The model under review builds one solid part; all positions refer to its coordinate system, in mm. A direction names the side the tool comes from. Coordinates: 2 decimals unless noted, no trailing zeros. Write each loop counter-clockwise with the first axis right and the second up, starting at its lowest first coordinate (ties: lowest second). Pieces come first, ordered by that corner, then holes. Notation, with made-up numbers: M 1,32 L 59,32 A23 cw 59,48 Z; hole C 43.25,6.5 d9. An arc over 180 degrees is marked long. Answer as a JSON object with one key per item and string values.
```python
from build123d import *

# Parameters (mm, degrees)
F0_W          = 310
F0_H          = 200
F1_DEPTH      = 15
F3_R          = 10
F2_R          = 6.5
F4_DEPTH      = 4
F4_DEPTH_BACK = 1
F5_R          = 6.5
F6_DEPTH      = 4
F6_DEPTH_BACK = 1


with BuildPart() as f1:
    # F0 (on Front) → F1 (new body)
    with BuildSketch(Plane.XZ):
        Rectangle(F0_W, F0_H)
    extrude(amount=F1_DEPTH)

    # F3
    f3_edges = [f1.edges().sort_by_distance(p)[0] for p in [
        (0, 0, -100),
    ]]
    fillet(f3_edges, radius=F3_R)

    # F2 (on face) → F4 (join, two sides)
    with BuildSketch(Plane.YZ.offset(155)) as f4_sk:
        with BuildLine():
            Line((-26, -100), (-15, -100))
            Line((-15, -100), (-15, -73))
            Line((-15, -73), (-26, -73))
            ThreePointArc((-26, -73), (-39.5, -86.5), (-26, -100))
        make_face()
        with Locations((-26, -86.5)):
            Circle(F2_R, mode=Mode.SUBTRACT)
    extrude(amount=F4_DEPTH)
    extrude(f4_sk.sketch, amount=-F4_DEPTH_BACK)

    # F5 (on face) → F6 (join, two sides)
    with BuildSketch(Plane(origin=(-155, 0, 0), x_dir=(0, -1, 0), z_dir=(-1, 0, 0))) as f6_sk:
        with BuildLine():
            Line((26, -73), (15, -73))
            Line((15, -73), (15, -100))
            Line((15, -100), (26, -100))
            ThreePointArc((26, -100), (39.5, -86.5), (26, -73))
        make_face()
        with Locations((26, -86.5)):
            Circle(F5_R, mode=Mode.SUBTRACT)
    extrude(amount=F6_DEPTH)
    extrude(f6_sk.sketch, amount=-F6_DEPTH_BACK)


solid = f1.part
```
(1) Add section B-B on z = 69. Give the boundary of the cut face in (x, y).
Results list:
{"outline": "M -155,-15 L 155,-15 L 155,0 L -155,0 Z"}
(2) Add section A-A on x = 109.5. Give the boundary of the cut face in (y, z).
Results list:
{"outline": "M -15,-100 L -10,-100 A10 ccw 0,-90 L 0,100 L -15,100 Z"}
(3) Draft analysis for pull direction X (two halves, no side actions). For faces 3 (the face through (159, -33, -86)), 4 (the face through (-159, -33, -86)), 5 (the face through (154, -33, -86)), state which applies: released by +X, released by -X, zero draft, split by the parting line, or undercut.
Results list:
{"face 3": "released by +X", "face 4": "released by -X", "face 5": "undercut"}
(4) Wall thickness on line 1 along Z through (x, y) = (154.2, -26); line 2 along X through (y, z) = (-30.5, -76.5); line 3 along Y through (x, z) = (-107.5, 24): over which ranges is each line inside the solid? List them lowest first. Write a range as from..to.
Results list:
{"line 1": "-100..-93, -80..-73", "line 2": "-159..-154, 154..159", "line 3": "-15..0"}
(5) For faces 1 (the face through (-154, -33, -86)), 2 (the face through (-156.535, -39.497, -86.797)), list the 3-axis set-ups (+Z, -Z, +X, -X, +Y, -Y) from which the entire face can be reached by the end or side of a thin tool; tool diameter is ignored.
Results list:
{"face 1": "+Z, -Z, -Y", "face 2": "+X, -X, -Y"}
(6) For pin 1 Ø1.5 at (x, y) = (84, -17.5) entering from -Z; pin 2 Ø4 at (x, z) = (-70.5, -43.5) entering from -Y; pin 3 Ø3 at (x, z) = (-157, -87) entering from +Y; pin 4 Ø4.5 at (y, z) = (-5.5, -40) entering from -X, all flat-tipped, find the tip position at first contact; note any pin that passes through.
Results list:
{"pin 1": "through", "pin 2": "y = -15", "pin 3": "y = -15", "pin 4": "x = -155"}
